Design review of the part shown in the three views and the two pictorial views. Dimensions are in mm from the part's minimum x, y and z. A direction names the side the tool comes from. Coordinates: 2 decimals unless noted, no trailing zeros. Loops run counter-clockwise (first coordinate to the right, second up) from the corner with the lowest first, then second, coordinate; pieces in that order, holes last. Notation, with made-up numbers: M 42.25,-2.5 L 79.25,-2.5 A12 cw 79.25,10.5 Z; hole C 59.25,80 d2. An arc over 180 degrees is marked long. Use one line per item in the form item = value.
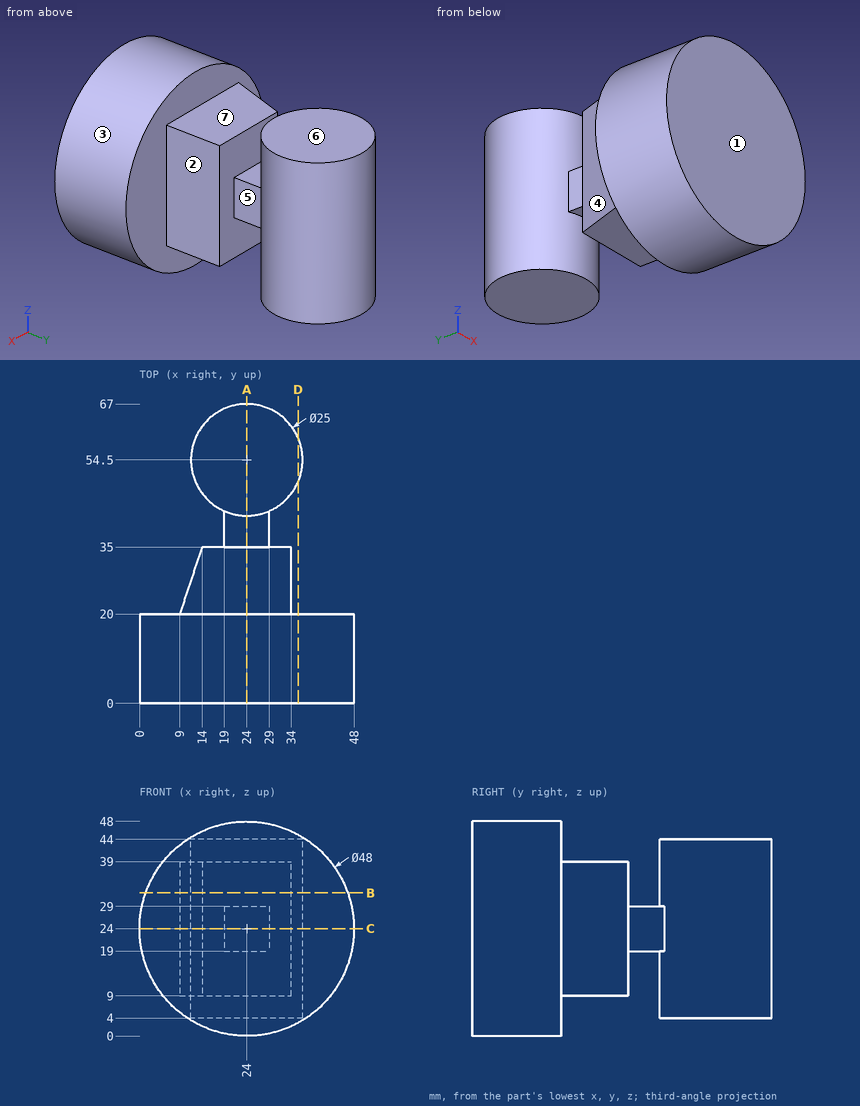
1. Add section C-C (z = 24). State the section outline as (x, y) points.
Response values:
outline = M 0,0 L 48,0 L 48,20 L 34,20 L 34,35 L 29,35 L 29,43.04 A12.5 ccw long 19,43.04 L 19,35 L 14,35 L 9,20 L 0,20 Z
2. Add section D-D (x = 35.5). State the section outline as (y, z) points, then the cut area to 3 significant figures.
Response values:
outline = M 0,2.93 L 20,2.93 L 20,45.07 L 0,45.07 Z; M 49.6,4 L 59.4,4 L 59.4,44 L 49.6,44 Z
area = 1,230 mm^2
3. Insertion check: P1, Ø8, axis at y = 30, z = 42, coming from the +X side; P2, Ø6, axis at x = 34.5, z = 40, coming from the +Y side; P3, Ø12.5, axis at x = 22.5, y = 58, coming from the -Z side; P4, Ø16, axis at x = 19, z = 20, coming from the +Y side. Each pin has a flat end and moves straight along its axis. Give the tip position at first contact, or say it passes through.
Response values:
P1 = 34
P2 = 64.5
P3 = 4
P4 = 67
4. Add section A-A (x = 24). State the section outline as (y, z) points.
Response values:
outline = M 0,0 L 20,0 L 20,9 L 35,9 L 35,19 L 42,19 L 42,4 L 67,4 L 67,44 L 42,44 L 42,29 L 35,29 L 35,39 L 20,39 L 20,48 L 0,48 Z
5. The part is to be moulded in two halves that separate along Y. For the marked faces 1, 2 and 3, say which applies: pulls with the +Y half, pulls with the -Y half, needs draft (parallel to the pull), parting line crosses it, or undercut.
Response values:
face_1 = pulls with the -Y half
face_2 = undercut
face_3 = needs draft
6. Machinability: for the marked faces 4, 5, 6 and 7, which of the approach directions +Z, -Z, +X, -X, +Y, -Y give a long, thin tool a straight path to every point of the face, cutting with its end or side? Answer none if there is none.
Response values:
face_4 = +Z, -Z, -X
face_5 = +Z, -Z, +X
face_6 = +Z, +X, -X, +Y
face_7 = +Z, +X, -X
7. Wall thickness on line 1 along Y through (x, z) = (24, 32); line 2 along Y through (x, z) = (3.5, 12); line 3 along Y through (x, z) = (17, 16.5): over which ranges is each line inside the solid? List them lowest first. Write a range as from..to.
Response values:
line_1 = 0..35, 42..67
line_2 = 0..20
line_3 = 0..35, 44.14..64.86
8. Add section B-B (z = 32). State the section outline as (x, y) points, then the cut area to 3 significant figures.
Response values:
outline = M 1.37,0 L 46.63,0 L 46.63,20 L 34,20 L 34,35 L 14,35 L 9,20 L 1.37,20 Z; C 24,54.5 d25
area = 1,730 mm^2
